from build123d import *

# Parameters (mm, degrees)
SKETCH1_W               = 20
SKETCH1_H               = 20
SKETCH1_W_2             = 17.6
SKETCH1_H_2             = 17.6
BOSS_EXTRUDE1_DEPTH     = 650
CUT_EXTRUDE1_DEPTH      = 1
CUT_EXTRUDE1_DEPTH_BACK = 21
CUT_EXTRUDE3_DEPTH      = 1
CUT_EXTRUDE3_DEPTH_BACK = 21


with BuildPart() as part:
    # Sketch1 → Boss-Extrude1 (new body)
    with BuildSketch(Plane(origin=(0, 0, 0), x_dir=(0, 0, -1), z_dir=(1, 0, 0))):
        Rectangle(SKETCH1_W, SKETCH1_H)
        Rectangle(SKETCH1_W_2, SKETCH1_H_2, mode=Mode.SUBTRACT)
    extrude(amount=BOSS_EXTRUDE1_DEPTH)

    # Sketch2 → Cut-Extrude1 (cut, two sides)
    with BuildSketch(Plane(origin=(0, 0, -10), x_dir=(-1, 0, 0), z_dir=(0, 0, -1))) as cut_extrude1_sk:
        Polygon((926.744923045, 936.744923045), (0, 10), (-20, -10), (-946.744923045, -936.744923045), (906.744923045, -2790.234769136), (2780.234769136, -916.744923045), align=None)
    extrude(amount=CUT_EXTRUDE1_DEPTH, mode=Mode.SUBTRACT)
    extrude(cut_extrude1_sk.sketch, amount=-CUT_EXTRUDE1_DEPTH_BACK, mode=Mode.SUBTRACT)

    # Sketch3 → Cut-Extrude3 (cut, two sides)
    with BuildSketch(Plane(origin=(0, 0, -10), x_dir=(-1, 0, 0), z_dir=(0, 0, -1))) as cut_extrude3_sk:
        Polygon((-1576.744923045, 936.744923045), (-650, 10), (-630, -10), (296.744923045, -936.744923045), (-1556.744923045, -2790.234769136), (-3430.234769136, -916.744923045), align=None)
    extrude(amount=CUT_EXTRUDE3_DEPTH, mode=Mode.SUBTRACT)
    extrude(cut_extrude3_sk.sketch, amount=-CUT_EXTRUDE3_DEPTH_BACK, mode=Mode.SUBTRACT)


solid = part.part
Can you work these out from the model? Positions are in its coordinate system, mm. A direction names the side the tool comes from. Coordinates: 2 decimals unless noted, no trailing zeros. Loops run counter-clockwise (first coordinate to the right, second up) from the corner with the lowest first, then second, coordinate; pieces in that order, holes last. Notation, with made-up numbers: (-19.75, 79.25) - (0.25, 79.25) arc R32 cw to (0.25, 112.25) - close; hole circle Ø9 at (2, 23). An arc over 180 degrees is marked (long way). Answer as a JSON object with one key per item and string values. Group by question number.
Item 1: If we mould it in two halves opening along Z, with no side actions, what happens to faces 1 (the face through (320, 10, 0)), 2 (the face through (320, 0, 10)), 3 (the face through (321, -8.8, 0))? For each: released by +Z, released by -Z, zero draft, split by the parting line, or undercut.
Item 2: If we section it at B-B (x = 410.5): List the corners of the cut face in (y, z) for me.
Item 3: If we section it at A-A (y = 1.5): List the corners of the cut face in (x, z) for me, plus the area to 3 significant figures.
Item 4: If I drill on L1, parallel to Z at x = 188, y = -1.5, over which ranges is the centre line in solid material (lowest first)? Write a range as from..to.
Item 5: For pin 1 (12 mm diameter, centred on y = -3.5, z = -3.5, fed in from -X); pin 2 (12 mm diameter, centred on y = 2.5, z = 3.5, fed in from -X), each with a flat end and sliding along its axis, tell me the tip position at first contact or that it passes through.
Item 6: If we section it at C-C (z = 5.5): List the corners of the cut face in (x, y) for me, plus the area to 3 significant figures.
Item 7: On a 3-axis mill with a long thin cutter (end or side, diameter ignored), from which of +Z, -Z, +X, -X, +Y, -Y can I reach the whole of each face in a straight line? I mean faces 4 (the face through (321, -10, 0)), 5 (the face through (320, 8.8, 0)). Say none if no direction works.
Returned:
{
 "1": {"face 1": "zero draft", "face 2": "released by +Z", "face 3": "undercut"},
 "2": {"outline": "(-10, -10) - (10, -10) - (10, 10) - (-10, 10) - close; hole (-8.8, -8.8) - (8.8, -8.8) - (8.8, 8.8) - (-8.8, 8.8) - close"},
 "3": {"outline": "(8.5, -10) - (641.5, -10) - (641.5, -8.8) - (8.5, -8.8) - close; (8.5, 8.8) - (641.5, 8.8) - (641.5, 10) - (8.5, 10) - close", "area": "1,520 mm²"},
 "4": {"L1": "z = -10..-8.8, 8.8..10"},
 "5": {"pin 1": "stops at x = 10.69", "pin 2": "stops at x = 4.69"},
 "6": {"outline": "(0, 10) - (1.2, 8.8) - (648.8, 8.8) - (650, 10) - close; (18.8, -8.8) - (20, -10) - (630, -10) - (631.2, -8.8) - close", "area": "1,510 mm²"},
 "7": {"face 4": "+Z, -Z, +X, -X, -Y", "face 5": "+X, -X"}
}
